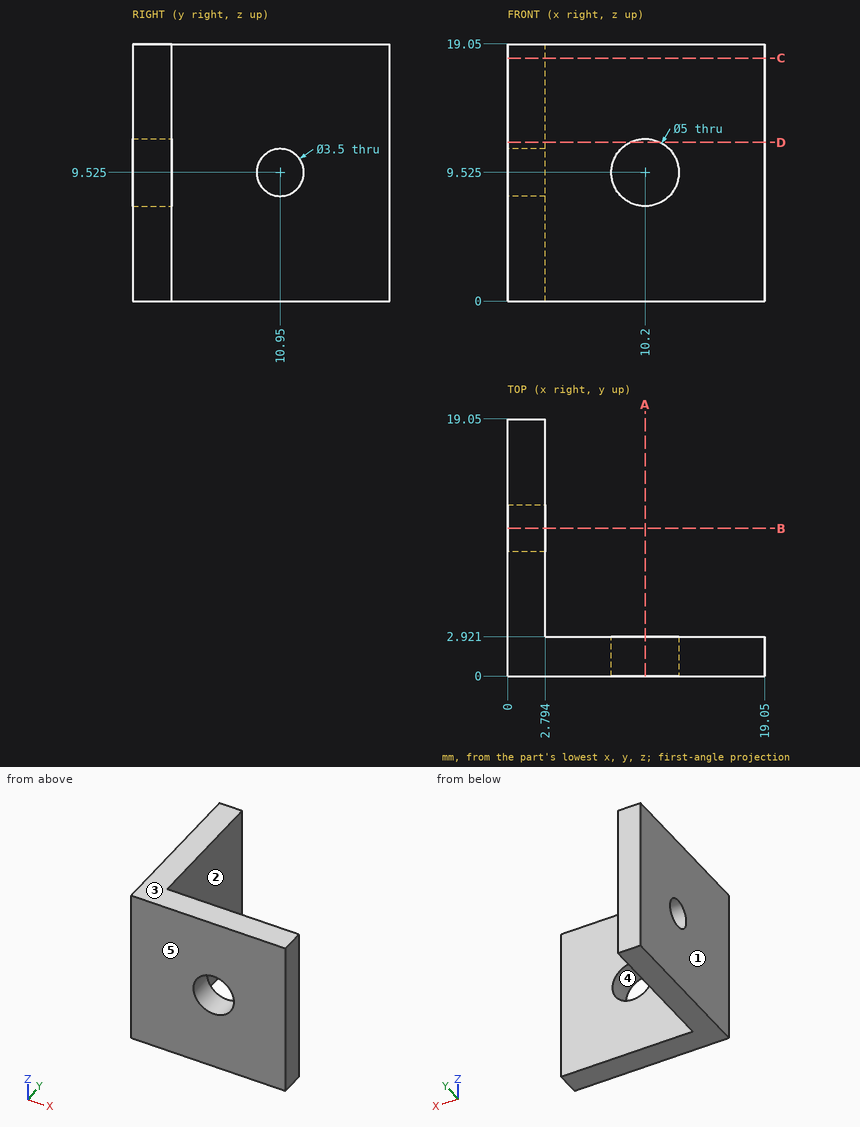
Input: dimensioned drawing with shaded views. Units: mm. Origin: part minimum x, y, z. A direction names the side the tool comes from. Round coordinates to 2 decimals unless told otherwise and drop trailing zeros. Loops run counter-clockwise (first coordinate to the right, second up) from the corner with the lowest first, then second, coordinate; pieces in that order, holes last. Notation, with made-up numbers: (10.25, -26.75) -> (63.25, -26.75) arc R16 cw to (63.25, -15.75) -> close; hole circle Ø8 at (61, 13.5). An arc over 180 degrees is marked (long way). Use one line per item in the form item = value. Start each with the question number.
1) Section A-A on x = 10.2. Output: boundary loops of the cut face in (y, z) (3 decimals), then the cut area to 3 significant figures.
2) Section C-C on z = 18. Output: boundary loops of the cut face in (x, y).
3) Draft query along Z for the marked faces 3, 4 and 5. Return one class per face: released by +Z, released by -Z, zero draft, split by the parting line, or undercut.
4) First-contact query: P1, Ø6, axis at y = 6.5, z = 3.5, coming from the +X side; P2, Ø4, axis at x = 11.5, z = 6.5, coming from the +Y side. Flat tips, straight axial feed; report the tip coordinate or a pass-through.
5) Section D-D on z = 11.75. Output: boundary loops of the cut face in (x, y), then the cut area to 4 significant figures.
6) Section B-B on y = 10.95. Output: boundary loops of the cut face in (x, z) (3 decimals).
7) Line query: L1, parallel to Z at x = 1, y = 10.95 (3 decimals); L2, parallel to Y at x = 15.5, z = 10.75; L3, parallel to Z at x = 10.2, y = 0.95 (3 decimals). Output: solid intervals per line, ascending.
8) Access query for the marked faces 1 and 2. Directions: +Z, -Z, +X, -X, +Y, -Y. A direction counts if a zero-diameter tool reaches every point of the face in a straight line with its end or side. Return the directions, or none.
Response:
q1.outline = (0, 0) -> (2.921, 0) -> (2.921, 7.025) -> (0, 7.025) -> close; (0, 12.025) -> (2.921, 12.025) -> (2.921, 19.05) -> (0, 19.05) -> close
q1.area = 41.0 mm^2
q2.outline = (0, 0) -> (19.05, 0) -> (19.05, 2.92) -> (2.79, 2.92) -> (2.79, 19.05) -> (0, 19.05) -> close
q3.face_3 = released by +Z
q3.face_4 = undercut
q3.face_5 = zero draft
q4.P1 = 2.79
q4.P2 = 2.92
q5.outline = (0, 0) -> (9.06, 0) -> (9.06, 2.92) -> (2.79, 2.92) -> (2.79, 19.05) -> (0, 19.05) -> close; (11.34, 0) -> (19.05, 0) -> (19.05, 2.92) -> (11.34, 2.92) -> close
q5.area = 94.05 mm^2
q6.outline = (0, 0) -> (2.794, 0) -> (2.794, 7.775) -> (0, 7.775) -> close; (0, 11.275) -> (2.794, 11.275) -> (2.794, 19.05) -> (0, 19.05) -> close
q7.L1 = 0 to 7.775, 11.275 to 19.05
q7.L2 = 0 to 2.92
q7.L3 = 0 to 7.025, 12.025 to 19.05
q8.face_1 = +Z, -Z, -X, +Y, -Y
q8.face_2 = +Z, -Z, +X, +Y
